Could you check a few things on this model? Use its own coordinates, in mm. Face numbers are marked on the shaded views. A direction names the side the tool comes from. Coordinates: 2 decimals unless noted, no trailing zeros. Order: outer loops, then holes, each group sorted by start corner. A loop starts at its lowest first (then second) coordinate and runs counter-clockwise, first axis right, second up. Notation, with made-up numbers: (4.5, 18) - (47.5, 18) arc R12 ccw to (47.5, 23) - close; hole circle Ø1 at (1, -32). An arc over 180 degrees is marked (long way). One line per item, written item: value.
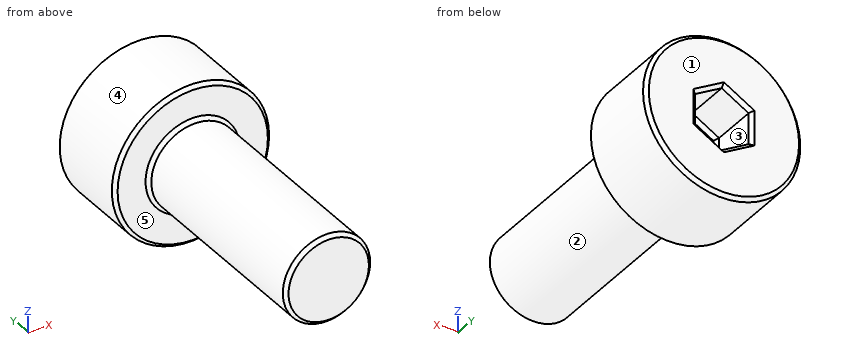
Autodesk Inventor part; units mm, degrees
ref_plane "YZ Plane" through (0, 0, 0) normal (1, 0, 0) x (0, 1, 0)
ref_plane "XZ Plane" through (0, 0, 0) normal (0, 1, 0) x (-1, 0, 0)
ref_plane "XY Plane" through (0, 0, 0) normal (0, 0, 1) x (1, 0, 0)
sketch "Sketch1" plane through (0, 0, 0) normal (0, 0, 1) x (1, 0, 0)
  line L0 (0, 8.5) -> (2.25, 8.5)
  line L1 (2.25, 8.5) -> (2.25, 6)
  line L2 (2.25, 6) -> (1.25, 6)
  line L3 (1.25, 6) -> (1.25, 0)
  line L4 (1.25, 0) -> (0, 0)
  line L5 (0, 0) -> (0, 8.5)
  dimension "d0" = 2.25
  dimension "d1" = 2.5
  dimension "d2" = 6
  dimension "d3" = 1.25
revolve "Revolution1" add sketch "Sketch1" angle 360 about axis through (0, 0, 0) along (0, 1, 0)
thread "Thread1"
sketch "Sketch3" plane through (0, 8.5, 0) normal (0, 1, 0) x (1, 0, 0)
  line L0 (0.77, -0.4446) -> (0, -0.8891)
  line L1 (0, -0.8891) -> (-0.77, -0.4446)
  line L2 (-0.77, -0.4446) -> (-0.77, 0.4446)
  line L3 (-0.77, 0.4446) -> (0, 0.8891)
  line L4 (0, 0.8891) -> (0.77, 0.4446)
  line L5 (0.77, 0.4446) -> (0.77, -0.4446)
  point P0 (0, 0)
  point P1 (0, 0)
  dimension "d13" = 1.54
extrude "Extrusion2" cut sketch "Sketch3" against normal blind 1.5
chamfer "Chamfer2" distance 0.1 angle 45 16 edges at (0.385, 8.5, 0.6668) (0.77, 8.5, 0) (0.77, 7, 0) (0.385, 8.5, -0.6668) (0.385, 7, -0.6668) (-0.385, 8.5, -0.6668) (-0.385, 7, -0.6668) (-0.77, 7, 0) (-0.77, 8.5, 0) (-0.385, 7, 0.6668) (-0.385, 8.5, 0.6668) (0.385, 7, 0.6668) (-2.25, 8.5, 0) (-2.25, 6, 0) (-1.25, 6, 0) (-1.25, 0, 0)
properties part number "M2.5 X 6"
Item 1: For the marked faces 1 and 2, which set-ups out of +Z, -Z, +X, -X, +Y, -Y let a thin tool reach every point of the face, with its end or its side?
Conclusion:
face 1: +Z, -Z, +X, -X, +Y
face 2: -Y
Item 2: Thinking about a two-plate mould opening in X: for the marked faces 3, 4 and 5, which applies, pulls with the +X half, pulls with the -X half, needs draft (parallel to the pull), parting line crosses it, or undercut?
Conclusion:
face 3: undercut
face 4: parting line crosses it
face 5: needs draft
Item 3: I'm going to push flat-ended pins straight in: pin 1 Ø1.3 at (x, z) = (0.5, 0.5) entering from -Y; pin 2 Ø2 at (y, z) = (6, 1.5) entering from -X. Where does each tip first touch, or does it pass through?
Conclusion:
pin 1: y = 0
pin 2: x = -2.19
Item 4: If I drill on probe 1 along Y at (x, z) = (-0.1, 0.2); probe 2 along Y at (x, z) = (-0.95, -1.1); probe 3 along X at (y, z) = (0.5, 0.9), over which ranges is the centre line in solid material (lowest first)?
Conclusion:
probe 1: 0 to 7
probe 2: 6 to 8.5
probe 3: -0.87 to 0.87
Item 5: I want a section at A-A on z = 0. Please give me the cut outline in (x, y).
Conclusion:
outline: (-2.25, 6.1) - (-2.15, 6) - (-1.35, 6) - (-1.25, 5.9) - (-1.25, 0.1) - (-1.15, 0) - (1.15, 0) - (1.25, 0.1) - (1.25, 5.9) - (1.35, 6) - (2.15, 6) - (2.25, 6.1) - (2.25, 8.4) - (2.15, 8.5) - (0.87, 8.5) - (0.77, 8.4) - (0.77, 7.1) - (0.67, 7) - (-0.67, 7) - (-0.77, 7.1) - (-0.77, 8.4) - (-0.87, 8.5) - (-2.15, 8.5) - (-2.25, 8.4) - close
Item 6: I want a section at B-B on y = 4.25. Please give me the cut outline in (x, z).
Conclusion:
outline: circle Ø2.5 at (0, 0)
